The listing builds one solid part. Answer for the finished solid, in the listing's coordinates (mm). A direction names the side the tool comes from. Round coordinates to 2 decimals unless told otherwise and drop trailing zeros. Order: outer loops, then holes, each group sorted by start corner. A loop starts at its lowest first (then second) coordinate and runs counter-clockwise, first axis right, second up. Notation, with made-up numbers: M -17,58 L 1,58 A17 cw 1,91 Z; hole C 40,4.5 d10. An arc over 180 degrees is marked long. Put each result on its own line as item: value. Start each with the question number.
1. The part is cut by section A-A (x = 10.5). Give the vertices of the cut face in (y, z), then the cut area to 3 significant figures.
2. The part is cut by section B-B (z = -5). Give the vertices of the cut face in (x, y).
3. The part is cut by section D-D (x = 5). Give the vertices of the cut face in (y, z), then the cut area to 3 significant figures.
4. The part is cut by section C-C (y = 20.75). Give the vertices of the cut face in (x, z), then the cut area to 3 significant figures.
5. Consider line 1 (X direction, y = -1.25, z = -16); line 2 (X direction, y = 28, z = -38.1); line 3 (Z direction, x = 5, y = -0.9). Determine where each line is inside the solid, lowest interval first.
6. Which of the six approach directions +Z, -Z, +X, -X, +Y, -Y give full straight-line access (tool end or side, diameter ignored) to faces 1 (the face through (14.5, -1.97, -5.07)), 2 (the face through (10, 16, -36))?
7. The mould has two halves that part along X. Classify faces 3 (the face through (10, -4, -20)), 4 (the face through (6.386, -1.972, -15.425)), 5 (the face through (21, -1, -29)): +X half, -X half, draft (parallel to the pull), parting line (faces both ways), or undercut.
8. Each of these flat-tipped pins is pushed along its axis until it touches: pin 1 Ø12 at (y, z) = (31, -28.5) entering from +X; pin 2 Ø1 at (x, y) = (7, 29) entering from +Z; pin 3 Ø8 at (x, z) = (7, -18.5) entering from +Y; pin 4 Ø5 at (x, z) = (16, -5) entering from -Y. Where does it stop, or does it pass through?
Autodesk Inventor part; units mm, degrees
ref_plane "YZ Plane" through (0, 0, 0) normal (1, 0, 0) x (0, 1, 0)
ref_plane "XZ Plane" through (0, 0, 0) normal (0, 1, 0) x (-1, 0, 0)
ref_plane "XY Plane" through (0, 0, 0) normal (0, 0, 1) x (1, 0, 0)
sketch "Sketch1" plane through (0, 0, 0) normal (1, 0, 0) x (0, 1, 0)
  line L0 (0, 0) -> (0, -36)
  line L1 (0, -36) -> (38, -36)
  line L2 (0, 0) -> (-4, 0)
  line L3 (-4, 0) -> (-4, -40)
  line L4 (-4, -40) -> (38, -40)
  line L5 (38, -40) -> (38, -36)
  dimension "d0" = 36
  dimension "d1" = 38
  dimension "d2" = 4
  dimension "d3" = 40
extrude "Extrusion1" add sketch "Sketch1" along normal blind 21
fillet "Fillet1" radius 10 2 edges at (21, 38, -38) (0, 38, -38)
sketch "Sketch2" plane through (0, 0, -36) normal (0, 0, 1) x (1, 0, 0)
  arc A0 (10, 38) -> (0, 28) centre (10, 28) ccw
  line L0 (0, 28) -> (21, 28)
  line L1 (0, 28) -> (0, 0)
  line L2 (0, 28) -> (10.5, 28)
  circle A1 centre (10.5, 28) radius 8
  circle A2 centre (10.5, 28) radius 6.5
  line L3 (4, 28) -> (2.5, 28)
  circle A3 centre (3.25, 28) radius 1.1
  line L4 (17, 28) -> (18.5, 28)
  circle A4 centre (17.75, 28) radius 1.1
  line L5 (10.5, 28) -> (10.5, 36)
  line L6 (10.5, 28) -> (10.5, 20)
  line L7 (10.5, 36) -> (10.5, 34.5)
  line L8 (10.5, 20) -> (10.5, 21.5)
  circle A5 centre (10.5, 35.25) radius 1.1
  circle A6 centre (10.5, 20.75) radius 1.1
  circle A7 centre (10.5, 28) radius 3
  dimension "d7" = 10.5
  dimension "d8" = 16
  dimension "d9" = 13
  dimension "d10" = 2.2
  dimension "d11" = 2.2
  dimension "d12" = 2.2
  dimension "d13" = 2.2
  dimension "d14" = 6
extrude "Extrusion2" cut sketch "Sketch2" against normal blind 21 contours A2 A3 A1 L0 | A2 A3 L0 | L0 A1 A3 A2 | L0 A3 A2 | A1 A3 L0 | L0 A3 A1 | A7 L5 L0 | L0 L6 A7 | A5 A1 L5 A2 | A2 L5 A5 | A6 L6 A2 | A2 L6 A1 A6 | A5 A1 | A1 A6 | L5 A7 L0 | L0 A7 L6 | L5 A1 A5 A2 | A2 A5 L5 | L6 A6 A2 | A2 A6 A1 L6 | A4 L0 A1 | A1 L0 A2 A4 | A4 A2 L0 A1 | A1 L0 A4 | A4 A2 L0 | L0 A2 A4
sketch "Sketch3" plane through (0, 0, 0) normal (0, 1, 0) x (1, 0, 0)
  line L0 (0, 36) -> (0, 0)
  line L1 (0, 0) -> (5, 0)
  line L2 (5, 0) -> (5, 5)
  line L3 (5, 5) -> (0, 5)
  line L4 (0, 5) -> (0, 0)
  line L5 (5, 5) -> (16, 5)
  line L6 (16, 5) -> (16, 16)
  line L7 (16, 16) -> (5, 16)
  line L8 (5, 16) -> (5, 5)
  circle A0 centre (5, 5) radius 1.5
  circle A1 centre (5, 16) radius 1.5
  circle A2 centre (16, 5) radius 1.5
  circle A3 centre (16, 16) radius 1.5
  dimension "d17" = 5
  dimension "d18" = 5
  dimension "d19" = 11
  dimension "d20" = 11
  dimension "d21" = 3
  dimension "d22" = 3
  dimension "d23" = 3
  dimension "d24" = 3
extrude "Extrusion3" cut sketch "Sketch3" against normal blind 21 contours A0 L8 L3 | L3 L2 A0 | L5 A0 L2 | L8 A0 L5 | A1 L7 L8 | L8 L7 A1 | A2 L6 L5 | L5 L6 A2 | A3 L6 L7 | L7 L6 A3
fillet "Fillet2" radius 3 1 edges at (10.5, 0, -36)
properties part number "L1"
Resolved:
1. outline: M -4,-40 L 19.65,-40 L 19.65,-36 L 3,-36 A3 cw 0,-33 L 0,0 L -4,0 Z; M 21.85,-40 L 25,-40 L 25,-36 L 21.85,-36 Z; M 31,-40 L 34.15,-40 L 34.15,-36 L 31,-36 Z; M 36.35,-40 L 38,-40 L 38,-36 L 36.35,-36 Z
1. area: 272 mm2
2. outline: M 0,-4 L 3.5,-4 L 3.5,0 L 0,0 Z; M 6.5,-4 L 14.5,-4 L 14.5,0 L 6.5,0 Z; M 17.5,-4 L 21,-4 L 21,0 L 17.5,0 Z
3. outline: M -4,-40 L 36.66,-40 L 36.66,-36 L 3,-36 A3 cw 0,-33 L 0,-17.5 L -4,-17.5 Z; M -4,-14.5 L 0,-14.5 L 0,-6.5 L -4,-6.5 Z; M -4,-3.5 L 0,-3.5 L 0,0 L -4,0 Z
3. area: 285 mm2
4. outline: M 0,-40 L 9.4,-40 L 9.4,-36 L 0,-36 Z; M 11.6,-40 L 21,-40 L 21,-36 L 11.6,-36 Z
4. area: 75.2 mm2
5. line 1: 0 to 3.5, 6.5 to 14.5, 17.5 to 21
5. line 2: 0 to 2.15, 4.35 to 7.5, 13.5 to 16.65, 18.85 to 21
5. line 3: -40 to -17.5, -14.5 to -6.5, -3.5 to 0
6. face 1: +Y, -Y
6. face 2: +Z, +X, -X, +Y
7. face 3: draft
7. face 4: undercut
7. face 5: +X half
8. pin 1: through
8. pin 2: z = -36
8. pin 3: y = 0
8. pin 4: y = -4
